from build123d import *

# Parameters (mm, degrees)
SKETCH_1_W                   = 40
SKETCH_1_H                   = 66.7
EXTRUDE_1_DEPTH              = 2
SKETCH_2_W                   = 4
SKETCH_2_H                   = 66.7
EXTRUDE_2_DEPTH              = 100
CUT_EXTRUDE_1_DEPTH          = 115.526077816
CUT_EXTRUDE_1_DEPTH_BACK     = 115.526077816
HOLE_WIZARD_M4_1_D           = 3.3
HOLE_WIZARD_M4_1_CSINK_D     = 4.05
HOLE_WIZARD_M4_1_CSINK_ANGLE = 90
HOLE_WIZARD_M4_2_AT_2_COUNT  = 2
HOLE_WIZARD_M4_2_AT_2_PITCH  = 68.59294731
HOLE_WIZARD_M4_2_AT_3_COUNT  = 2
HOLE_WIZARD_M4_2_AT_3_PITCH  = 26
HOLE_WIZARD_M4_2_AT_4_COUNT  = 2
HOLE_WIZARD_M4_2_AT_4_PITCH  = 62.376998966
HOLE_WIZARD_M4_2_AT_5_COUNT  = 2
HOLE_WIZARD_M4_2_AT_5_PITCH  = 56.7
SKETCH_11_W                  = 66.7
SKETCH_11_H                  = 2
EXTRUDE_3_DEPTH              = 100
SKETCH_13_W                  = 40
SKETCH_13_H                  = 66.7
EXTRUDE_4_DEPTH              = 2
SKETCH_14_W                  = 4
SKETCH_14_H                  = 66.7
EXTRUDE_5_DEPTH              = 100
CUT_EXTRUDE_2_DEPTH          = 180.589037806
CUT_EXTRUDE_2_DEPTH_BACK     = 180.589037806
HOLE_WIZARD_M4_3_AT_2_COUNT  = 2
HOLE_WIZARD_M4_3_AT_2_PITCH  = 26
HOLE_WIZARD_M4_3_AT_3_COUNT  = 2
HOLE_WIZARD_M4_3_AT_3_PITCH  = 62.376998966
HOLE_WIZARD_M4_3_AT_4_COUNT  = 2
HOLE_WIZARD_M4_3_AT_4_PITCH  = 56.7
CUT_EXTRUDE_3_REACH          = 181.589
SKETCH_18_R                  = 9.5
CUT_EXTRUDE_4_REACH          = 181.589
SKETCH_21_R                  = 11
CUT_EXTRUDE_5_REACH          = 181.589
SKETCH_22_R                  = 4.5
FILLET_1_R                   = 2
CUT_EXTRUDE_6_REACH          = 193.604
SKETCH_23_W                  = 36
SKETCH_23_H                  = 66.7
CUT_EXTRUDE_7_REACH          = 164.752
SKETCH_24_W                  = 36
SKETCH_24_H                  = 66.7
HOLE_START                   = -124
HOLE_WIZARD_M3_1_OUTLINE_R   = 1.25
HOLE_WIZARD_M3_1_DEPTH       = 4
CUT_EXTRUDE_8_DEPTH          = 154.990981879
CUT_EXTRUDE_8_DEPTH_BACK     = 154.990981879
SKETCH_27_W                  = 104
SKETCH_27_H                  = 66.7
FILLET_2_R                   = 0.8


# Read off the part's stored shape, not the designer's step: the hole wizard step, the hole wizard step
with BuildPart() as part:
    # Sketch 1 → Extrude 1 (new body)
    with BuildSketch(Plane(origin=(0, 0, 0), x_dir=(1, 0, 0), z_dir=(0, 1, 0))):
        Rectangle(SKETCH_1_W, SKETCH_1_H)
    extrude(amount=EXTRUDE_1_DEPTH)

    # Sketch 2 → Extrude 2 (add)
    with BuildSketch(Plane(origin=(0, 2, 0), x_dir=(1, 0, 0), z_dir=(0, 1, 0))):
        with Locations((-18, 0)):
            Rectangle(SKETCH_2_W, SKETCH_2_H)
    extrude(amount=EXTRUDE_2_DEPTH)

    # Sketch 5 → Cut-Extrude 1 (cut, two sides: drawn at the far end of the back side and taken through both)
    with BuildSketch(Plane.ZY.offset(20).offset(-CUT_EXTRUDE_1_DEPTH_BACK)):
        with BuildLine():
            ThreePointArc((0, 102), (23.582011153, 92.232011153), (33.35, 68.65))
            Line((33.35, 68.65), (33.35, 102))
            Line((33.35, 102), (0, 102))
        make_face()
        with BuildLine():
            ThreePointArc((-33.35, 68.65), (-23.582011153, 92.232011153), (0, 102))
            Line((0, 102), (-33.35, 102))
            Line((-33.35, 102), (-33.35, 68.65))
        make_face()
    extrude(amount=CUT_EXTRUDE_1_DEPTH + CUT_EXTRUDE_1_DEPTH_BACK, mode=Mode.SUBTRACT)

    # Hole Wizard M4 _1 (through all)
    with Locations(Plane.ZY.offset(20)):
        with Locations((0, 97.65), (25.11473671, 54.15), (-25.11473671, 54.15)):
            CounterSinkHole(HOLE_WIZARD_M4_1_D / 2, HOLE_WIZARD_M4_1_CSINK_D / 2, counter_sink_angle=HOLE_WIZARD_M4_1_CSINK_ANGLE)

    # Sketch 10 → Hole Wizard M4 _2 (revolve, cut)
    with BuildSketch(Plane(origin=(15, 2, -28.35), x_dir=(0, 0, 1), z_dir=(1, 0, 0))):
        Polygon((0, 0), (0, 2), (1.65, 2), (1.65, 0.375), (2.025, 0), align=None)
    hole_wizard_m4_2 = revolve(axis=Axis((15, 8.35, -28.35), (0, -1, 0)), mode=Mode.SUBTRACT)

    # Hole Wizard M4 _2 at 2: Hole Wizard M4 _2 ×2
    with Locations(*[Vector(-0.9508085645250022, 0, 0.3097790722852413) * (i * HOLE_WIZARD_M4_2_AT_2_PITCH) for i in range(1, HOLE_WIZARD_M4_2_AT_2_COUNT)]):
        add(hole_wizard_m4_2, mode=Mode.SUBTRACT)

    # Hole Wizard M4 _2 at 3: Hole Wizard M4 _2 ×2
    with Locations(*[(-i * HOLE_WIZARD_M4_2_AT_3_PITCH, 0, 0) for i in range(1, HOLE_WIZARD_M4_2_AT_3_COUNT)]):
        add(hole_wizard_m4_2, mode=Mode.SUBTRACT)

    # Hole Wizard M4 _2 at 4: Hole Wizard M4 _2 ×2
    with Locations(*[Vector(-0.4168203092647413, 0, 0.9089889052042635) * (i * HOLE_WIZARD_M4_2_AT_4_PITCH) for i in range(1, HOLE_WIZARD_M4_2_AT_4_COUNT)]):
        add(hole_wizard_m4_2, mode=Mode.SUBTRACT)

    # Hole Wizard M4 _2 at 5: Hole Wizard M4 _2 ×2
    with Locations(*[(0, 0, i * HOLE_WIZARD_M4_2_AT_5_PITCH) for i in range(1, HOLE_WIZARD_M4_2_AT_5_COUNT)]):
        add(hole_wizard_m4_2, mode=Mode.SUBTRACT)

    # Sketch 11 → Extrude 3 (add)
    with BuildSketch(Plane.ZY.offset(20)):
        with Locations((0, 16)):
            Rectangle(SKETCH_11_W, SKETCH_11_H)
    extrude(amount=EXTRUDE_3_DEPTH)



with BuildPart() as body_2:
    # Sketch 13 → Extrude 4 (new body)
    with BuildSketch(Plane(origin=(0, 0, 0), x_dir=(1, 0, 0), z_dir=(0, 1, 0))):
        with Locations((-140, 0)):
            Rectangle(SKETCH_13_W, SKETCH_13_H)
    extrude(amount=EXTRUDE_4_DEPTH)


with BuildPart() as part_1:
    add(part.part)

    add(body_2.part)  # Extrude 5 merges body 2
    # Sketch 14 → Extrude 5 (add)
    with BuildSketch(Plane(origin=(0, 2, 0), x_dir=(1, 0, 0), z_dir=(0, 1, 0))):
        with Locations((-122, 0)):
            Rectangle(SKETCH_14_W, SKETCH_14_H)
    extrude(amount=EXTRUDE_5_DEPTH)

    # Sketch 15 → Cut-Extrude 2 (cut, two sides: drawn at the far end of the back side and taken through both)
    with BuildSketch(Plane.ZY.offset(124).offset(-CUT_EXTRUDE_2_DEPTH_BACK)):
        with BuildLine():
            ThreePointArc((0, 102), (23.582011153, 92.232011153), (33.35, 68.65))
            Line((33.35, 68.65), (33.35, 102))
            Line((33.35, 102), (0, 102))
        make_face()
        with BuildLine():
            ThreePointArc((-33.35, 68.65), (-23.582011153, 92.232011153), (0, 102))
            Line((0, 102), (-33.35, 102))
            Line((-33.35, 102), (-33.35, 68.65))
        make_face()
    extrude(amount=CUT_EXTRUDE_2_DEPTH + CUT_EXTRUDE_2_DEPTH_BACK, mode=Mode.SUBTRACT)

    # Sketch 17 → Hole Wizard M4 _3 (revolve, cut)
    with BuildSketch(Plane(origin=(-129, 2, -28.35), x_dir=(0, 0, 1), z_dir=(1, 0, 0))):
        Polygon((0, 0), (0, 2), (1.65, 2), (1.65, 0.375), (2.025, 0), align=None)
    hole_wizard_m4_3 = revolve(axis=Axis((-129, 8.35, -28.35), (0, -1, 0)), mode=Mode.SUBTRACT)

    # Hole Wizard M4 _3 at 2: Hole Wizard M4 _3 ×2
    with Locations(*[(-i * HOLE_WIZARD_M4_3_AT_2_PITCH, 0, 0) for i in range(1, HOLE_WIZARD_M4_3_AT_2_COUNT)]):
        add(hole_wizard_m4_3, mode=Mode.SUBTRACT)

    # Hole Wizard M4 _3 at 3: Hole Wizard M4 _3 ×2
    with Locations(*[Vector(-0.41682030926474106, 0, 0.9089889052042636) * (i * HOLE_WIZARD_M4_3_AT_3_PITCH) for i in range(1, HOLE_WIZARD_M4_3_AT_3_COUNT)]):
        add(hole_wizard_m4_3, mode=Mode.SUBTRACT)

    # Hole Wizard M4 _3 at 4: Hole Wizard M4 _3 ×2
    with Locations(*[(0, 0, i * HOLE_WIZARD_M4_3_AT_4_PITCH) for i in range(1, HOLE_WIZARD_M4_3_AT_4_COUNT)]):
        add(hole_wizard_m4_3, mode=Mode.SUBTRACT)

    # Sketch 18 → Cut-Extrude 3 (cut, up to next)
    with BuildSketch(Plane.ZY.offset(124), mode=Mode.PRIVATE) as cut_extrude_3_sk1:
        with Locations((0, 68.65)):
            Circle(SKETCH_18_R)
    cut_extrude_3_tool1 = extrude(cut_extrude_3_sk1.sketch, amount=-CUT_EXTRUDE_3_REACH, mode=Mode.PRIVATE) & part_1.part
    add(cut_extrude_3_tool1.solids().sort_by_distance((-124, 68.65, 0))[0], mode=Mode.SUBTRACT)

    # Sketch 21 → Cut-Extrude 4 (cut, up to next)
    with BuildSketch(Plane(origin=(-16, 0, 0), x_dir=(0, 0, -1), z_dir=(1, 0, 0)), mode=Mode.PRIVATE) as cut_extrude_4_sk1:
        with Locations((0, 68.65)):
            Circle(SKETCH_21_R)
    cut_extrude_4_tool1 = extrude(cut_extrude_4_sk1.sketch, amount=-CUT_EXTRUDE_4_REACH, mode=Mode.PRIVATE) & part_1.part
    add(cut_extrude_4_tool1.solids().sort_by_distance((-16, 68.65, 0))[0], mode=Mode.SUBTRACT)

    # Sketch 22 → Cut-Extrude 5 (cut, up to next)
    with BuildSketch(Plane(origin=(-16, 0, 0), x_dir=(0, 0, -1), z_dir=(1, 0, 0)), mode=Mode.PRIVATE) as cut_extrude_5_sk1:
        with Locations((16.670989023, 59.025)):
            Circle(SKETCH_22_R)
    cut_extrude_5_tool1 = extrude(cut_extrude_5_sk1.sketch, amount=-CUT_EXTRUDE_5_REACH, mode=Mode.PRIVATE) & part_1.part
    add(cut_extrude_5_tool1.solids().sort_by_distance((-16, 59.025, -16.670989))[0], mode=Mode.SUBTRACT)

    # Fillet 1
    fillet_1_edges = [part_1.edges().sort_by_distance(p)[0] for p in [
        (-160, 1, -33.35),
        (-160, 1, 33.35),
        (20, 1, 33.35),
        (20, 1, -33.35),
    ]]
    fillet(fillet_1_edges, radius=FILLET_1_R)

    # Sketch 23 → Cut-Extrude 6 (cut, up to next)
    with BuildSketch(Plane(origin=(0, 2, 0), x_dir=(1, 0, 0), z_dir=(0, 1, 0)), mode=Mode.PRIVATE) as cut_extrude_6_sk1:
        with Locations((-142, 0)):
            Rectangle(SKETCH_23_W, SKETCH_23_H)
    cut_extrude_6_tool1 = extrude(cut_extrude_6_sk1.sketch, amount=-CUT_EXTRUDE_6_REACH, mode=Mode.PRIVATE) & part_1.part
    add(cut_extrude_6_tool1.solids().sort_by_distance((-142, 2, 0))[0], mode=Mode.SUBTRACT)

    # Sketch 24 → Cut-Extrude 7 (cut, up to next)
    with BuildSketch(Plane(origin=(0, 2, 0), x_dir=(1, 0, 0), z_dir=(0, 1, 0)), mode=Mode.PRIVATE) as cut_extrude_7_sk1:
        with Locations((2, 0)):
            Rectangle(SKETCH_24_W, SKETCH_24_H)
    cut_extrude_7_tool1 = extrude(cut_extrude_7_sk1.sketch, amount=-CUT_EXTRUDE_7_REACH, mode=Mode.PRIVATE) & part_1.part
    add(cut_extrude_7_tool1.solids().sort_by_distance((2, 2, 0))[0], mode=Mode.SUBTRACT)

    # Hole Wizard M3 _1 outline → Hole Wizard M3 _1 (cut)
    with BuildSketch(Plane.YZ.offset(HOLE_START)):
        with Locations((6, -9)):
            Circle(HOLE_WIZARD_M3_1_OUTLINE_R)
        with Locations((6, 9)):
            Circle(HOLE_WIZARD_M3_1_OUTLINE_R)
    extrude(amount=HOLE_WIZARD_M3_1_DEPTH, mode=Mode.SUBTRACT)

    # Hole Wizard M3 _1 2 outline → Hole Wizard M3 _1 2 (revolve, cut)
    with BuildSketch(Plane(origin=(0, 6, -9), x_dir=(0, 1, 0), z_dir=(0, 0, -1))):
        Polygon((1.525, -16), (0, -16), (0, -20), (1.25, -20), (1.25, -16.275), align=None)
    revolve(axis=Axis((0, 6, -9), (1, 0, 0)), mode=Mode.SUBTRACT)

    # Hole Wizard M3 _1 3 outline → Hole Wizard M3 _1 3 (revolve, cut)
    with BuildSketch(Plane(origin=(0, 6, 9), x_dir=(0, 1, 0), z_dir=(0, 0, -1))):
        Polygon((0, -20), (1.25, -20), (1.25, -16.275), (1.525, -16), (0, -16), align=None)
    revolve(axis=Axis((0, 6, 9), (1, 0, 0)), mode=Mode.SUBTRACT)

    # Sketch 27 → Cut-Extrude 8 (cut, two sides: drawn at the far end of the back side and taken through both)
    with BuildSketch(Plane(origin=(0, 17, 0), x_dir=(1, 0, 0), z_dir=(0, 1, 0)).offset(-CUT_EXTRUDE_8_DEPTH_BACK)):
        with Locations((-72, 0)):
            Rectangle(SKETCH_27_W, SKETCH_27_H)
    extrude(amount=CUT_EXTRUDE_8_DEPTH + CUT_EXTRUDE_8_DEPTH_BACK, mode=Mode.SUBTRACT)

    # Hole Wizard M2.5 _1 outline → Hole Wizard M2.5 _1 (revolve, cut)
    with BuildSketch(Plane(origin=(0, 21, -9), x_dir=(0, 1, 0), z_dir=(0, 0, -1))):
        Polygon((1.025, -19.75), (1.025, -16), (0, -16), (0, -20), (1.275, -20), align=None)
    revolve(axis=Axis((0, 21, -9), (1, 0, 0)), mode=Mode.SUBTRACT)

    # Hole Wizard M2.5 _1 2 outline → Hole Wizard M2.5 _1 2 (revolve, cut)
    with BuildSketch(Plane(origin=(0, 21, 9), x_dir=(0, 1, 0), z_dir=(0, 0, -1))):
        Polygon((1.025, -19.75), (1.025, -16), (0, -16), (0, -20), (1.275, -20), align=None)
    revolve(axis=Axis((0, 21, 9), (1, 0, 0)), mode=Mode.SUBTRACT)

    # Fillet 2
    fillet_2_edges = [part_1.edges().sort_by_distance(p)[0] for p in [
        (-16, 34.325, -33.35),
        (-20, 34.325, -33.35),
        (-20, 102, 0),
        (-16, 102, 0),
        (-16, 34.325, 33.35),
        (-20, 34.325, 33.35),
        (-18, 0, 33.35),
    ]]
    fillet(fillet_2_edges, radius=FILLET_2_R)


solid = part_1.part
Design review of the part built by this model. Coordinates are the model's own, in mm. Coordinates: 2 decimals unless noted, no trailing zeros. Loops run counter-clockwise (first coordinate to the right, second up) from the corner with the lowest first, then second, coordinate; pieces in that order, holes last. Notation, with made-up numbers: M 51,-21 L 87,-21 A13 ccw 87,-15 Z; hole C 73.25,-36.75 d10. An arc over 180 degrees is marked long. Use one line per item in the form item = value.
(1) For line 1 along Z through (x, y) = (-18.1, 54.15); line 2 along Z through (x, y) = (-17.9, 21) (3 decimals); line 3 along Z through (x, y) = (-17.35, 65.5), list the stretches that pass through material, from the lowest coordinate up. Write a range as from..to.
Return value:
line_1 = -33.35..-26.76, -23.46..23.46, 26.76..33.35
line_2 = -33.35..-10.025, -7.975..7.975, 10.025..33.35
line_3 = -33.35..-10.54, 10.54..33.35
(2) Clearance check with flat-ended pins moving along their axes: P1, Ø2.5, axis at y = 21, z = -9, coming from the -X side (3 decimals); P2, Ø3, axis at y = 6, z = -9, coming from the +X side (3 decimals). State where each tip first meets the part, or that it passes through.
Return value:
P1 = -19.975
P2 = -16.025
(3) Draft analysis for pull direction Z (two halves, no side actions). For faces 1 (the face through (-18, 34, -33.35)), 2 (the face through (-17.97, 57.91, 2.38)), 3 (the face through (-17.787, 53.146, 26.424)), 4 (the face through (-18, 0, -1)), state which applies: pulls with the +Z half, pulls with the -Z half, needs draft (parallel to the pull), parting line crosses it, or undercut.
Return value:
face_1 = pulls with the -Z half
face_2 = undercut
face_3 = undercut
face_4 = needs draft
(4) Consider section A-A (y = 21). Write out the cut boundary in (x, z) (3 decimals).
Return value:
outline = M -20,-32.55 A0.8 ccw -19.2,-33.35 L -16.8,-33.35 A0.8 ccw -16,-32.55 L -16,-10.025 L -19.75,-10.025 L -20,-10.275 Z; M -20,-7.725 L -19.75,-7.975 L -16,-7.975 L -16,7.975 L -19.75,7.975 L -20,7.725 Z; M -20,10.275 L -19.75,10.025 L -16,10.025 L -16,32.55 A0.8 ccw -16.8,33.35 L -19.2,33.35 A0.8 ccw -20,32.55 Z
(5) Consider section B-B (x = -17.9). Give the number of separate pieces and of enclosed holes in the cut face, and give its area (3 significant figures).
Return value:
separate_pieces = 1
enclosed_holes = 9
area = 5,840 mm2
(6) Consider section C-C (y = 6). Write out the cut boundary in (x, z) (3 decimals), and give its area (3 significant figures).
Return value:
outline = M -20,-32.55 A0.8 ccw -19.2,-33.35 L -16.8,-33.35 A0.8 ccw -16,-32.55 L -16,-10.525 L -16.275,-10.25 L -20,-10.25 Z; M -20,-7.75 L -16.275,-7.75 L -16,-7.475 L -16,7.475 L -16.275,7.75 L -20,7.75 Z; M -20,10.25 L -16.275,10.25 L -16,10.525 L -16,32.55 A0.8 ccw -16.8,33.35 L -19.2,33.35 A0.8 ccw -20,32.55 Z
area = 246 mm2
